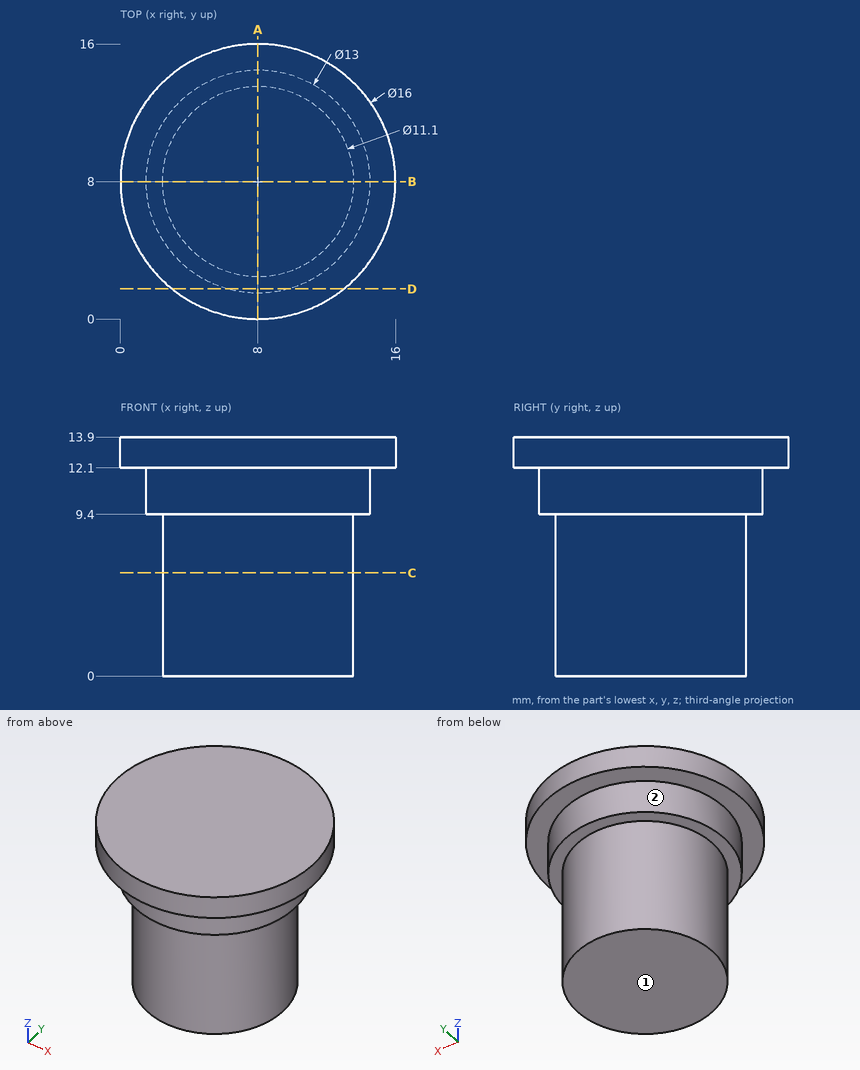
Input: dimensioned drawing with shaded views. Units: mm. Origin: part minimum x, y, z. A direction names the side the tool comes from. Give positions to 0.01 mm unless a question says otherwise; leave off trailing zeros. Order: outer loops, then holes, each group sorted by start corner. A loop starts at its lowest first (then second) coordinate and runs counter-clockwise, first axis right, second up. Notation, with made-up numbers: (-10, -5.75) -> (44, -5.75) arc R25 ccw to (44, 11.25) -> close; hole circle Ø10 at (68.5, 35.5). An arc over 180 degrees is marked (long way). Use a Markdown table: item, result.
1) Section query C-C, the plane z = 6. Return the cut outline in (x, y), then the cut area to 3 significant figures.
Answer list:
| item | result |
|---|---|
| outline | circle Ø11.1 at (8, 8) |
| area | 96.8 mm² |
2) Section query A-A, the plane x = 8. Return the cut outline in (y, z).
Answer list:
| item | result |
|---|---|
| outline | (0, 12.1) -> (1.5, 12.1) -> (1.5, 9.4) -> (2.45, 9.4) -> (2.45, 0) -> (13.55, 0) -> (13.55, 9.4) -> (14.5, 9.4) -> (14.5, 12.1) -> (16, 12.1) -> (16, 13.9) -> (0, 13.9) -> close |
3) Contact query for flat-ended pins moving along their axis: P1, Ø2, axis at x = 7, z = 2, coming from the -Y side; P2, Ø3, axis at y = 13, z = 11, coming from the -X side; P3, Ø4, axis at x = 7.5, z = 11.5, coming from the +Y side; P4, Ø1.5, axis at x = 1.5, y = 8.5, coming from the -Z side. Output: stop coordinate, or through.
Answer list:
| item | result |
|---|---|
| P1 | y = 2.45 |
| P2 | x = 1.06 |
| P3 | y = 16 |
| P4 | z = 9.4 |
4) Section query D-D, the plane y = 1.75. Return the cut outline in (x, z), then the cut area to 3 significant figures.
Answer list:
| item | result |
|---|---|
| outline | (3.01, 12.1) -> (6.21, 12.1) -> (6.21, 9.4) -> (9.79, 9.4) -> (9.79, 12.1) -> (12.99, 12.1) -> (12.99, 13.9) -> (3.01, 13.9) -> close |
| area | 27.6 mm² |
5) Reachability of the marked faces 1 and 2 from +Z, -Z, +X, -X, +Y, -Y: full face, straight path, thin tool, end or side. Return the list, or none.
Answer list:
| item | result |
|---|---|
| face 1 | -Z, +X, -X, +Y, -Y |
| face 2 | -Z |
6) Ray query, line 1 along Z through (x, y) = (3.5, 11.5); line 2 along Y through (x, z) = (7.75, 2.5); line 3 along Z through (x, y) = (1.5, 12.5). Return the intervals inside material, ascending. Write a range as [from, to].
Answer list:
| item | result |
|---|---|
| line 1 | [9.4, 13.9] |
| line 2 | [2.46, 13.54] |
| line 3 | [12.1, 13.9] |
